```python
from build123d import *

# Parameters (mm, degrees)
SKETCH1_W                 = 120
SKETCH1_H                 = 120
BOSS_EXTRUDE1_DEPTH       = 2.7
CUT_EXTRUDE1_REACH        = 171.727
SKETCH2_W                 = 13.492346384
SKETCH2_H                 = 25
SKETCH2_W_2               = 14.089535058
SKETCH2_3_W               = 30
SKETCH2_3_H               = 12
BOSS_EXTRUDE2_DEPTH       = 16
CUT_EXTRUDE2_REACH        = 169.256
SKETCH4_R                 = 3.5
CUT_EXTRUDE3_REACH        = 169.256
SKETCH5_R                 = 3.5
CUT_EXTRUDE4_REACH        = 172.458
SKETCH6_R                 = 2.5
BOSS_EXTRUDE4_START       = 56
BOSS_EXTRUDE4_OUTLINE_W   = 1
BOSS_EXTRUDE4_OUTLINE_H   = 24
BOSS_EXTRUDE4_DEPTH       = 8.5
BOSS_EXTRUDE5_START       = -39
BOSS_EXTRUDE5_OUTLINE_W   = 2.5
BOSS_EXTRUDE5_OUTLINE_H   = 10
BOSS_EXTRUDE5_OUTLINE_W_2 = 3
BOSS_EXTRUDE5_DEPTH       = 27
BOSS_EXTRUDE5_START_2     = -15
BOSS_EXTRUDE5_2_OUTLINE_W = 8.5
BOSS_EXTRUDE5_2_OUTLINE_H = 10
BOSS_EXTRUDE5_2_DEPTH     = 3
CUT_EXTRUDE5_REACH        = 172.458
SKETCH8_W                 = 13.93792073
SKETCH8_H                 = 24.444968664
SKETCH8_W_2               = 11.364766133
SKETCH8_H_2               = 21.442954969
SKETCH8_W_3               = 15.276468839
SKETCH8_H_3               = 17.022275105
SKETCH8_H_4               = 21.442954968
SKETCH8_W_4               = 15.490753693
SKETCH9_W                 = 5
SKETCH9_H                 = 5
BOSS_EXTRUDE6_DEPTH       = 32
SKETCH10_W                = 6
SKETCH10_H                = 6
BOSS_EXTRUDE7_DEPTH       = 48


# Read off the part's stored shape, not the designer's step: Boss-Extrude4, Boss-Extrude5
with BuildPart() as part:
    # Sketch1 → Boss-Extrude1 (new body)
    with BuildSketch(Plane(origin=(0, 0, 0), x_dir=(1, 0, 0), z_dir=(0, 1, 0))):
        with Locations((60, 60)):
            Rectangle(SKETCH1_W, SKETCH1_H)
    extrude(amount=BOSS_EXTRUDE1_DEPTH)

    # Sketch2 → Cut-Extrude1 (cut, up to next)
    with BuildSketch(Plane(origin=(0, 2.7, 0), x_dir=(1, 0, 0), z_dir=(0, 1, 0)), mode=Mode.PRIVATE) as cut_extrude1_sk1:
        with Locations((46.746173192, 97.5)):
            Rectangle(SKETCH2_W, SKETCH2_H)
    cut_extrude1_tool1 = extrude(cut_extrude1_sk1.sketch, amount=-CUT_EXTRUDE1_REACH, mode=Mode.PRIVATE) & part.part
    # Sketch2 → Cut-Extrude1 (cut, up to next)
    with BuildSketch(Plane(origin=(0, 2.7, 0), x_dir=(1, 0, 0), z_dir=(0, 1, 0)), mode=Mode.PRIVATE) as cut_extrude1_sk2:
        with Locations((72.955232471, 97.5)):
            Rectangle(SKETCH2_W_2, SKETCH2_H)
    cut_extrude1_tool2 = extrude(cut_extrude1_sk2.sketch, amount=-CUT_EXTRUDE1_REACH, mode=Mode.PRIVATE) & part.part
    add(cut_extrude1_tool1.solids().sort_by_distance((46.746173, 2.7, -97.5))[0], mode=Mode.SUBTRACT)
    add(cut_extrude1_tool2.solids().sort_by_distance((72.955232, 2.7, -97.5))[0], mode=Mode.SUBTRACT)

    # Sketch2<3> → Boss-Extrude2 (add)
    with BuildSketch(Plane(origin=(0, 2.7, 0), x_dir=(1, 0, 0), z_dir=(0, 1, 0))):
        with Locations((20, 113)):
            Rectangle(SKETCH2_3_W, SKETCH2_3_H)
        with Locations((100, 113)):
            Rectangle(SKETCH2_3_W, SKETCH2_3_H)
    extrude(amount=BOSS_EXTRUDE2_DEPTH)

    # Sketch4 → Cut-Extrude2 (cut, up to next)
    with BuildSketch(Plane.ZY.offset(-5), mode=Mode.PRIVATE) as cut_extrude2_sk1:
        with Locations((-113, 12.7)):
            Circle(SKETCH4_R)
    cut_extrude2_tool1 = extrude(cut_extrude2_sk1.sketch, amount=-CUT_EXTRUDE2_REACH, mode=Mode.PRIVATE) & part.part
    add(cut_extrude2_tool1.solids().sort_by_distance((5, 12.7, -113))[0], mode=Mode.SUBTRACT)

    # Sketch5 → Cut-Extrude3 (cut, up to next)
    with BuildSketch(Plane(origin=(115, 0, 0), x_dir=(0, 0, -1), z_dir=(1, 0, 0)), mode=Mode.PRIVATE) as cut_extrude3_sk1:
        with Locations(Location((113, 12.7, 0), (0, 0, 180))):
            Circle(SKETCH5_R)
    cut_extrude3_tool1 = extrude(cut_extrude3_sk1.sketch, amount=-CUT_EXTRUDE3_REACH, mode=Mode.PRIVATE) & part.part
    add(cut_extrude3_tool1.solids().sort_by_distance((115, 12.7, -113))[0], mode=Mode.SUBTRACT)

    # Sketch6 → Cut-Extrude4 (cut, up to next)
    with BuildSketch(Plane(origin=(0, 2.7, 0), x_dir=(1, 0, 0), z_dir=(0, 1, 0)), mode=Mode.PRIVATE) as cut_extrude4_sk1:
        with Locations(Location((7, 13, 0), (0, 0, 270))):
            Circle(SKETCH6_R)
    cut_extrude4_tool1 = extrude(cut_extrude4_sk1.sketch, amount=-CUT_EXTRUDE4_REACH, mode=Mode.PRIVATE) & part.part
    # Sketch6 → Cut-Extrude4 (cut, up to next)
    with BuildSketch(Plane(origin=(0, 2.7, 0), x_dir=(1, 0, 0), z_dir=(0, 1, 0)), mode=Mode.PRIVATE) as cut_extrude4_sk2:
        with Locations(Location((4.26, 51, 0), (0, 0, 270))):
            Circle(SKETCH6_R)
    cut_extrude4_tool2 = extrude(cut_extrude4_sk2.sketch, amount=-CUT_EXTRUDE4_REACH, mode=Mode.PRIVATE) & part.part
    # Sketch6 → Cut-Extrude4 (cut, up to next)
    with BuildSketch(Plane(origin=(0, 2.7, 0), x_dir=(1, 0, 0), z_dir=(0, 1, 0)), mode=Mode.PRIVATE) as cut_extrude4_sk3:
        with Locations(Location((37.96, 51, 0), (0, 0, 270))):
            Circle(SKETCH6_R)
    cut_extrude4_tool3 = extrude(cut_extrude4_sk3.sketch, amount=-CUT_EXTRUDE4_REACH, mode=Mode.PRIVATE) & part.part
    # Sketch6 → Cut-Extrude4 (cut, up to next)
    with BuildSketch(Plane(origin=(0, 2.7, 0), x_dir=(1, 0, 0), z_dir=(0, 1, 0)), mode=Mode.PRIVATE) as cut_extrude4_sk4:
        with Locations(Location((84.78, 13, 0), (0, 0, 270))):
            Circle(SKETCH6_R)
    cut_extrude4_tool4 = extrude(cut_extrude4_sk4.sketch, amount=-CUT_EXTRUDE4_REACH, mode=Mode.PRIVATE) & part.part
    # Sketch6 → Cut-Extrude4 (cut, up to next)
    with BuildSketch(Plane(origin=(0, 2.7, 0), x_dir=(1, 0, 0), z_dir=(0, 1, 0)), mode=Mode.PRIVATE) as cut_extrude4_sk5:
        with Locations(Location((82.04, 51, 0), (0, 0, 270))):
            Circle(SKETCH6_R)
    cut_extrude4_tool5 = extrude(cut_extrude4_sk5.sketch, amount=-CUT_EXTRUDE4_REACH, mode=Mode.PRIVATE) & part.part
    # Sketch6 → Cut-Extrude4 (cut, up to next)
    with BuildSketch(Plane(origin=(0, 2.7, 0), x_dir=(1, 0, 0), z_dir=(0, 1, 0)), mode=Mode.PRIVATE) as cut_extrude4_sk6:
        with Locations(Location((115.74, 51.20220141, 0), (0, 0, 270))):
            Circle(SKETCH6_R)
    cut_extrude4_tool6 = extrude(cut_extrude4_sk6.sketch, amount=-CUT_EXTRUDE4_REACH, mode=Mode.PRIVATE) & part.part
    # Sketch6 → Cut-Extrude4 (cut, up to next)
    with BuildSketch(Plane(origin=(0, 2.7, 0), x_dir=(1, 0, 0), z_dir=(0, 1, 0)), mode=Mode.PRIVATE) as cut_extrude4_sk7:
        with Locations(Location((113, 13, 0), (0, 0, 270))):
            Circle(SKETCH6_R)
    cut_extrude4_tool7 = extrude(cut_extrude4_sk7.sketch, amount=-CUT_EXTRUDE4_REACH, mode=Mode.PRIVATE) & part.part
    # Sketch6 → Cut-Extrude4 (cut, up to next)
    with BuildSketch(Plane(origin=(0, 2.7, 0), x_dir=(1, 0, 0), z_dir=(0, 1, 0)), mode=Mode.PRIVATE) as cut_extrude4_sk8:
        with Locations(Location((35.22, 13, 0), (0, 0, 270))):
            Circle(SKETCH6_R)
    cut_extrude4_tool8 = extrude(cut_extrude4_sk8.sketch, amount=-CUT_EXTRUDE4_REACH, mode=Mode.PRIVATE) & part.part
    add(cut_extrude4_tool1.solids().sort_by_distance((7, 2.7, -13))[0], mode=Mode.SUBTRACT)
    add(cut_extrude4_tool2.solids().sort_by_distance((4.26, 2.7, -51))[0], mode=Mode.SUBTRACT)
    add(cut_extrude4_tool3.solids().sort_by_distance((37.96, 2.7, -51))[0], mode=Mode.SUBTRACT)
    add(cut_extrude4_tool4.solids().sort_by_distance((84.78, 2.7, -13))[0], mode=Mode.SUBTRACT)
    add(cut_extrude4_tool5.solids().sort_by_distance((82.04, 2.7, -51))[0], mode=Mode.SUBTRACT)
    add(cut_extrude4_tool6.solids().sort_by_distance((115.74, 2.7, -51.202201))[0], mode=Mode.SUBTRACT)
    add(cut_extrude4_tool7.solids().sort_by_distance((113, 2.7, -13))[0], mode=Mode.SUBTRACT)
    add(cut_extrude4_tool8.solids().sort_by_distance((35.22, 2.7, -13))[0], mode=Mode.SUBTRACT)

    # Boss-Extrude4 outline → Boss-Extrude4 (add)
    with BuildSketch(Plane.YZ.offset(BOSS_EXTRUDE4_START)):
        with Locations((3.2, -27)):
            Rectangle(BOSS_EXTRUDE4_OUTLINE_W, BOSS_EXTRUDE4_OUTLINE_H)
    extrude(amount=BOSS_EXTRUDE4_DEPTH)

    # Boss-Extrude5 outline → Boss-Extrude5 (add)
    with BuildSketch(Plane.XY.offset(BOSS_EXTRUDE5_START)):
        with Locations((65.75, 7.7)):
            Rectangle(BOSS_EXTRUDE5_OUTLINE_W, BOSS_EXTRUDE5_OUTLINE_H)
        with Locations((54.5, 7.7)):
            Rectangle(BOSS_EXTRUDE5_OUTLINE_W_2, BOSS_EXTRUDE5_OUTLINE_H)
    extrude(amount=BOSS_EXTRUDE5_DEPTH)

    # Boss-Extrude5 2 outline → Boss-Extrude5 2 (add)
    with BuildSketch(Plane.XY.offset(BOSS_EXTRUDE5_START_2)):
        with Locations((60.25, 7.7)):
            Rectangle(BOSS_EXTRUDE5_2_OUTLINE_W, BOSS_EXTRUDE5_2_OUTLINE_H)
    extrude(amount=BOSS_EXTRUDE5_2_DEPTH)

    # Sketch8 → Cut-Extrude5 (cut, up to next)
    with BuildSketch(Plane(origin=(0, 2.7, 0), x_dir=(1, 0, 0), z_dir=(0, 1, 0)), mode=Mode.PRIVATE) as cut_extrude5_sk1:
        with Locations((99.838592928, 71.277482239)):
            Rectangle(SKETCH8_W, SKETCH8_H)
    cut_extrude5_tool1 = extrude(cut_extrude5_sk1.sketch, amount=-CUT_EXTRUDE5_REACH, mode=Mode.PRIVATE) & part.part
    # Sketch8 → Cut-Extrude5 (cut, up to next)
    with BuildSketch(Plane(origin=(0, 2.7, 0), x_dir=(1, 0, 0), z_dir=(0, 1, 0)), mode=Mode.PRIVATE) as cut_extrude5_sk2:
        with Locations((21.518433658, 33.503955022)):
            Rectangle(SKETCH8_W_2, SKETCH8_H_2)
    cut_extrude5_tool2 = extrude(cut_extrude5_sk2.sketch, amount=-CUT_EXTRUDE5_REACH, mode=Mode.PRIVATE) & part.part
    # Sketch8 → Cut-Extrude5 (cut, up to next)
    with BuildSketch(Plane(origin=(0, 2.7, 0), x_dir=(1, 0, 0), z_dir=(0, 1, 0)), mode=Mode.PRIVATE) as cut_extrude5_sk3:
        with Locations((20.660272656, 70.634411505)):
            Rectangle(SKETCH8_W, SKETCH8_H)
    cut_extrude5_tool3 = extrude(cut_extrude5_sk3.sketch, amount=-CUT_EXTRUDE5_REACH, mode=Mode.PRIVATE) & part.part
    # Sketch8 → Cut-Extrude5 (cut, up to next)
    with BuildSketch(Plane(origin=(0, 2.7, 0), x_dir=(1, 0, 0), z_dir=(0, 1, 0)), mode=Mode.PRIVATE) as cut_extrude5_sk4:
        with Locations((46.474954565, 69.366478605)):
            Rectangle(SKETCH8_W_3, SKETCH8_H_3)
    cut_extrude5_tool4 = extrude(cut_extrude5_sk4.sketch, amount=-CUT_EXTRUDE5_REACH, mode=Mode.PRIVATE) & part.part
    # Sketch8 → Cut-Extrude5 (cut, up to next)
    with BuildSketch(Plane(origin=(0, 2.7, 0), x_dir=(1, 0, 0), z_dir=(0, 1, 0)), mode=Mode.PRIVATE) as cut_extrude5_sk5:
        with Locations((99.705334599, 32.777682609)):
            Rectangle(SKETCH8_W_2, SKETCH8_H_4)
    cut_extrude5_tool5 = extrude(cut_extrude5_sk5.sketch, amount=-CUT_EXTRUDE5_REACH, mode=Mode.PRIVATE) & part.part
    # Sketch8 → Cut-Extrude5 (cut, up to next)
    with BuildSketch(Plane(origin=(0, 2.7, 0), x_dir=(1, 0, 0), z_dir=(0, 1, 0)), mode=Mode.PRIVATE) as cut_extrude5_sk6:
        with Locations((72.867080872, 69.52199516)):
            Rectangle(SKETCH8_W_4, SKETCH8_H_3)
    cut_extrude5_tool6 = extrude(cut_extrude5_sk6.sketch, amount=-CUT_EXTRUDE5_REACH, mode=Mode.PRIVATE) & part.part
    add(cut_extrude5_tool1.solids().sort_by_distance((99.838593, 2.7, -71.277482))[0], mode=Mode.SUBTRACT)
    add(cut_extrude5_tool2.solids().sort_by_distance((21.518434, 2.7, -33.503955))[0], mode=Mode.SUBTRACT)
    add(cut_extrude5_tool3.solids().sort_by_distance((20.660273, 2.7, -70.634412))[0], mode=Mode.SUBTRACT)
    add(cut_extrude5_tool4.solids().sort_by_distance((46.474955, 2.7, -69.366479))[0], mode=Mode.SUBTRACT)
    add(cut_extrude5_tool5.solids().sort_by_distance((99.705335, 2.7, -32.777683))[0], mode=Mode.SUBTRACT)
    add(cut_extrude5_tool6.solids().sort_by_distance((72.867081, 2.7, -69.521995))[0], mode=Mode.SUBTRACT)

    # Sketch9 → Boss-Extrude6 (add)
    with BuildSketch(Plane(origin=(0, 18.7, 0), x_dir=(1, 0, 0), z_dir=(0, 1, 0))):
        with Locations((20, 113)):
            Rectangle(SKETCH9_W, SKETCH9_H)
        with Locations((100, 113)):
            Rectangle(SKETCH9_W, SKETCH9_H)
    extrude(amount=BOSS_EXTRUDE6_DEPTH)

    # Sketch10 → Boss-Extrude7 (add)
    with BuildSketch(Plane(origin=(0, 2.7, 0), x_dir=(1, 0, 0), z_dir=(0, 1, 0))):
        with Locations((117, 3)):
            Rectangle(SKETCH10_W, SKETCH10_H)
        with Locations((3, 3)):
            Rectangle(SKETCH10_W, SKETCH10_H)
    extrude(amount=BOSS_EXTRUDE7_DEPTH)


solid = part.part
```
Part model, mm, in its own coordinate system. A direction names the side the tool comes from. Give positions to 0.01 mm unless a question says otherwise; leave off trailing zeros. Order: outer loops, then holes, each group sorted by start corner. A loop starts at its lowest first (then second) coordinate and runs counter-clockwise, first axis right, second up. Notation, with made-up numbers: (89.25, -34.75) - (106.25, -34.75) arc R32 ccw to (106.25, -5.75) - close; hole circle Ø4 at (-24, -13.5). An arc over 180 degrees is marked (long way). Use one line per item in the form item = value.
Item 1: Slice it at B-B on z = -67. Give the cut face in (x, y).
Solution:
outline = (0, 0) - (13.69, 0) - (13.69, 2.7) - (0, 2.7) - close; (27.63, 0) - (38.84, 0) - (38.84, 2.7) - (27.63, 2.7) - close; (54.11, 0) - (65.12, 0) - (65.12, 2.7) - (54.11, 2.7) - close; (80.61, 0) - (92.87, 0) - (92.87, 2.7) - (80.61, 2.7) - close; (106.81, 0) - (120, 0) - (120, 2.7) - (106.81, 2.7) - close
Item 2: Two-plate mould, pull along Z, no slides. Class faces 1 (the face through (100.21, 14.041, -109.767)), 2 (the face through (55, 12.7, -26)), 3 (the face through (40, 1, -97)), 4 (the face through (60, 8, -15)): released by +Z, released by -Z, zero draft, split by the parting line, or undercut.
Solution:
face_1 = undercut
face_2 = zero draft
face_3 = undercut
face_4 = released by -Z
Item 3: Slice it at A-A on y = 7. Give the cut face in (x, z).
Solution:
outline = (0, -6) - (6, -6) - (6, 0) - (0, 0) - close; (5, -119) - (35, -119) - (35, -107) - (5, -107) - close; (53, -39) - (56, -39) - (56, -15) - (64.5, -15) - (64.5, -39) - (67, -39) - (67, -12) - (53, -12) - close; (85, -119) - (115, -119) - (115, -107) - (85, -107) - close; (114, -6) - (120, -6) - (120, 0) - (114, 0) - close
Item 4: Pin check, flat tips, straight feed: pin 1 Ø2.5 at (y, z) = (35.5, -113.5) entering from +X; pin 2 Ø1 at (x, z) = (77.5, -34) entering from +Y; pin 3 Ø13 at (x, y) = (25.5, 13) entering from -Z; pin 4 Ø8 at (x, y) = (74.5, 14.5) entering from +Z. Stop position of each tip, or through.
Solution:
pin_1 = 102.5
pin_2 = 2.7
pin_3 = -119
pin_4 = through
Item 5: Which spindle directions (+Z, -Z, +X, -X, +Y, -Y) get a long thin tool onto all of the face, cutting with end or side? Do faces 5 (the face through (20, 50.7, -113)), 6 (the face through (80.612, 1, -69)), 7 (the face through (64.5, 8, -27)), 8 (the face through (102.5, 34, -113)), 9 (the face through (97.5, 34, -113)). Say none if no direction does.
Solution:
face_5 = +Z, -Z, +X, -X, +Y
face_6 = +Y, -Y
face_7 = -Z, +Y
face_8 = +Z, -Z, +X, +Y
face_9 = +Z, -Z, +Y
Item 6: Slice it at D-D on z = -102.5. Give the cut face in (x, y), and give its area (3 significant figures).
Solution:
outline = (0, 0) - (40, 0) - (40, 2.7) - (0, 2.7) - close; (53.49, 0) - (65.91, 0) - (65.91, 2.7) - (53.49, 2.7) - close; (80, 0) - (120, 0) - (120, 2.7) - (80, 2.7) - close
area = 250 mm2
Item 7: Probe probe 1 along X at (y, z) = (1, -13); probe 2 along X at (y, z) = (20, -4.5); probe 3 along X at (y, z) = (1, -51). List the from-to ranges inside material, lowest first. Write a range as from..to.
Solution:
probe_1 = 0..4.5, 9.5..32.72, 37.72..82.28, 87.28..110.5, 115.5..120
probe_2 = 0..6, 114..120
probe_3 = 0..1.76, 6.76..35.46, 40.46..79.54, 84.54..113.25, 118.23..120
Item 8: Slice it at C-C on x = 46. Give the cut face in (y, z), and give its area (3 significant figures).
Solution:
outline = (0, -120) - (2.7, -120) - (2.7, -110) - (0, -110) - close; (0, -85) - (2.7, -85) - (2.7, -77.88) - (0, -77.88) - close; (0, -60.86) - (2.7, -60.86) - (2.7, 0) - (0, 0) - close
area = 211 mm2
